CAD build for the part. Positions are in the model's coordinates, mm. Round coordinates to 2 decimals unless told otherwise and drop trailing zeros. Use one line per item in the form item = value. Start each with the question number.
Item 1: Pin check, flat tip, straight feed: pin 1 (2 mm diameter, centred on y = 0.5, z = 0.5, fed in from -X). Stop position of the tip, or through.
Item 2: Drill centre lines: L1, parallel to X at y = -0.75, z = 0.4; L2, parallel to Z at x = 2, y = 3; L3, parallel to Y at x = -2.25, z = 3.85. Where is each one in solid material? Low to high.
Item 3: Pull direction Y, two halves, no side cores. Call faces 1 (the flat face through (0, -5.779, 2)), 2 (the flat face through (0, 4.221, 2)), 3 (the flat face through (0, -1, 0)): +Y half, -Y half, draft (parallel to the pull), parting line (faces both ways), or undercut.
from build123d import *

# Parameters (mm, degrees)
BOSS_EXTRUDE1_DEPTH = 5
FILLET1_R           = 0.5


with BuildPart() as part:
    # Sketch1 → Boss-Extrude1 (new body)
    with BuildSketch(Plane.XY):
        with BuildLine():
            Line((-4.492753623, 3.605072464), (-4.492753623, 4.221014493))
            Line((-4.492753623, 4.221014493), (4.492753623, 4.221014493))
            Line((4.492753623, 4.221014493), (4.492753623, 3.605072464))
            add(Edge.make_bspline(
                [(4.456521739, -5.126811594), (-1.030105298, -4.776601358), (0.235507246, 3.605072464), (4.492753623, 3.605072464)],
                knots=[0, 0, 0, 0, 1, 1, 1, 1], degree=3))
            Line((4.456521739, -5.126811594), (4.456521739, -5.778985507))
            Line((4.456521739, -5.778985507), (-4.456521739, -5.778985507))
            Line((-4.456521739, -5.778985507), (-4.456521739, -5.126811594))
            add(Edge.make_bspline(
                [(-4.456521739, -5.126811594), (1.030105298, -4.776601358), (-0.235507246, 3.605072464), (-4.492753623, 3.605072464)],
                knots=[0, 0, 0, 0, 1, 1, 1, 1], degree=3))
        make_face()
    extrude(amount=BOSS_EXTRUDE1_DEPTH)

    # Fillet1
    fillet1_edges = [part.edges().sort_by_distance(p)[0] for p in [
        (-0.809667973, -0.814408993, 0),
        (-4.492753623, 3.605072464, 2.5),
        (4.492753623, 3.605072464, 2.5),
        (4.456521739, -5.126811594, 2.5),
        (-4.456521739, -5.126811594, 2.5),
        (0.809667973, -0.814408993, 5),
        (-0.809667973, -0.814408993, 5),
        (0.809667973, -0.814408993, 0),
    ]]
    fillet(fillet1_edges, radius=FILLET1_R)


solid = part.part
Determined:
q1.pin_1 = -1.41
q2.L1 = -0.8 to 0.8
q2.L2 = 0.01 to 4.99
q2.L3 = -5.78 to -4.35, 2.66 to 4.22
q3.face_1 = -Y half
q3.face_2 = +Y half
q3.face_3 = draft
